Print and shaded views of the part. All mm, measured from the part's lowest x, y and z. Give positions to 0.01 mm unless a question says otherwise; leave off trailing zeros. Order: outer loops, then holes, each group sorted by start corner. A loop starts at its lowest first (then second) coordinate and runs counter-clockwise, first axis right, second up. Notation, with made-up numbers: (73, 28.5) - (132, 28.5) arc R19 cw to (132, 60.5) - close; hole circle Ø2 at (56.5, -9.5). An arc over 180 degrees is marked (long way). Answer in a Markdown table with one row per item.
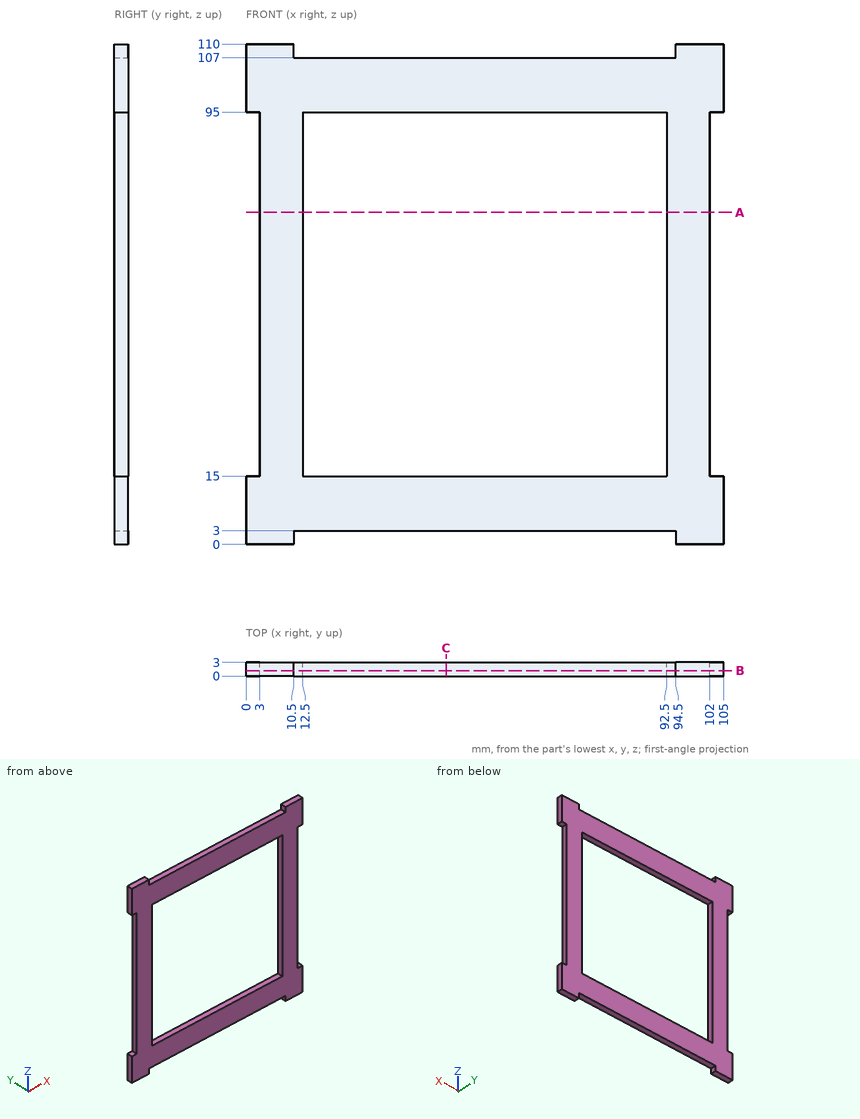
1. Cut at C-C on x = 44. Write the cut outline in (y, z).
Check result:
| item | result |
|---|---|
| outline | (0, 3) - (3, 3) - (3, 15) - (0, 15) - close; (0, 95) - (3, 95) - (3, 107) - (0, 107) - close |
2. Cut at A-A on z = 73. Write the cut outline in (x, y), and give its area (3 significant figures).
Check result:
| item | result |
|---|---|
| outline | (3, 0) - (12.5, 0) - (12.5, 3) - (3, 3) - close; (92.5, 0) - (102, 0) - (102, 3) - (92.5, 3) - close |
| area | 57.0 mm² |
3. Drop flat-ended pins along their axis: P1, Ø0.9, axis at x = 1.5, y = 1, coming from the -Z side; P2, Ø1, axis at x = 47, y = 0.5, coming from the -Z side; P3, Ø0.9, axis at x = 44.5, y = 1, coming from the +Z side; P4, Ø1.5, axis at y = 1.5, z = 40, coming from the +X side. Give the stop position or say it passes through.
Check result:
| item | result |
|---|---|
| P1 | stops at z = 0 |
| P2 | stops at z = 3 |
| P3 | stops at z = 107 |
| P4 | stops at x = 102 |
4. Cut at B-B on y = 1.2. Write the cut outline in (x, z), and give its area (3 significant figures).
Check result:
| item | result |
|---|---|
| outline | (0, 0) - (10.5, 0) - (10.5, 3) - (94.5, 3) - (94.5, 0) - (105, 0) - (105, 15) - (102, 15) - (102, 95) - (105, 95) - (105, 110) - (94.5, 110) - (94.5, 107) - (10.5, 107) - (10.5, 110) - (0, 110) - (0, 95) - (3, 95) - (3, 15) - (0, 15) - close; hole (12.5, 15) - (92.5, 15) - (92.5, 95) - (12.5, 95) - close |
| area | 4,170 mm² |
5. Probe line 1 (Z direction, x = 86, y = 2); line 2 (X direction, y = 1.1, z = 30.5). List the from-to ranges inside material, lowest first.
Check result:
| item | result |
|---|---|
| line 1 | z = 3 to 15, 95 to 107 |
| line 2 | x = 3 to 12.5, 92.5 to 102 |
